Autodesk Inventor part; units mm, degrees
ref_plane "YZ Plane" through (0, 0, 0) normal (1, 0, 0) x (0, 1, 0)
ref_plane "XZ Plane" through (0, 0, 0) normal (0, 1, 0) x (-1, 0, 0)
ref_plane "XY Plane" through (0, 0, 0) normal (0, 0, 1) x (1, 0, 0)
sketch "Sketch1" plane through (0, 0, 0) normal (0, 1, 0) x (-1, 0, 0)
  circle A0 centre (0, 0) radius 20.5
  dimension "d0" = 41
extrude "Extrusion1" add sketch "Sketch1" along normal blind 20
sketch "Sketch2" plane through (0, 20, 0) normal (0, 1, 0) x (1, 0, 0)
  circle A0 centre (0, 0) radius 20.5
  circle A1 centre (0, 0) radius 17.15
  dimension "d3" = 34.3
extrude "Extrusion2" add sketch "Sketch2" along normal blind 7 contours A1
sketch "Sketch3" plane through (0, 0, 0) normal (0, -1, 0) x (1, 0, 0)
  circle A0 centre (0, 0) radius 15
  circle A1 centre (0, 0) radius 12.8774
  dimension "d6" = 30
extrude "Extrusion3" add sketch "Sketch3" along normal blind 30
properties part number "100"
Could you check a few things on this model? Use its own coordinates, in mm. A direction names the side the tool comes from. Coordinates: 2 decimals unless noted, no trailing zeros. Write each loop counter-clockwise with the first axis right and the second up, starting at its lowest first coordinate (ties: lowest second). Pieces come first, ordered by that corner, then holes. Notation, with made-up numbers: (46.5, -34) -> (104.5, -34) arc R28 ccw to (104.5, -1) -> close; hole circle Ø8 at (-37.75, 60). An arc over 180 degrees is marked (long way). Write item = value, one per line. Start each with the question number.
(1) I need wall thicknesses on line 1 (Z direction, x = 0.5, y = -0.5); line 2 (Z direction, x = -11.5, y = -9); line 3 (Y direction, x = 9.5, z = 18). Which ranges of each line are inside material? Lowest first, please. Write a range as [from, to].
(2) Which directions (+Z, -Z, +X, -X, +Y, -Y) give clear straight access to the entire face, cutting with the end or side of a thin tool? Please do faces 4 (the face through (-2.79, -14.79, 12.57)), 5 (the face through (5, 20, -17)), 6 (the face through (4.444, 9.86, 20.013)).
(3) I want a section at B-B (x = 0). Please give me the cut outline in (y, z).
(4) Will these pins go through, and if not, where does the flat tip stop? pin 1 (6 mm diameter, centred on x = 4.5, y = -23.5, fed in from +Z); pin 2 (4 mm diameter, centred on x = -1.5, z = 3.5, fed in from -Y); pin 3 (3 mm diameter, centred on x = 4, y = 19.5, fed in from -Z).
(5) I want a section at C-C (y = -23.5). Please give me the cut outline in (x, z), plus the area to 3 significant figures.
(6) I want a section at D-D (y = 8.5). Please give me the cut outline in (x, z), plus the area to 3 significant figures.
(7) We'd pull the mould along X, two halves only. Please class faces 1 (the face through (-1.4, 0, -15.1)), 2 (the face through (0, 0, 0)), 3 (the face through (16.36, 23.45, 5.15)): released by +X, released by -X, zero draft, split by the parting line, or undercut.
(8) I want a section at A-A (z = 0). Please give me the cut outline in (x, y).
Result set:
q1.line_1 = [-14.99, -12.87], [12.87, 14.99]
q1.line_2 = [-9.63, -5.79], [5.79, 9.63]
q1.line_3 = [0, 20]
q2.face_4 = -Y
q2.face_5 = +Y
q2.face_6 = +Y, -Y
q3.outline = (-30, -15) -> (0, -15) -> (0, -20.5) -> (20, -20.5) -> (20, -17.15) -> (27, -17.15) -> (27, 17.15) -> (20, 17.15) -> (20, 20.5) -> (0, 20.5) -> (0, 15) -> (-30, 15) -> (-30, 12.88) -> (0, 12.88) -> (0, -12.88) -> (-30, -12.88) -> close
q4.pin_1 = 14.92
q4.pin_2 = 0
q4.pin_3 = -20.35
q5.outline = circle Ø30 at (0, 0); hole circle Ø25.75 at (0, 0)
q5.area = 186 mm2
q6.outline = circle Ø41 at (0, 0)
q6.area = 1,320 mm2
q7.face_1 = zero draft
q7.face_2 = undercut
q7.face_3 = split by the parting line
q8.outline = (-20.5, 0) -> (-15, 0) -> (-15, -30) -> (-12.88, -30) -> (-12.88, 0) -> (12.88, 0) -> (12.88, -30) -> (15, -30) -> (15, 0) -> (20.5, 0) -> (20.5, 20) -> (17.15, 20) -> (17.15, 27) -> (-17.15, 27) -> (-17.15, 20) -> (-20.5, 20) -> close
